Design review of the part built by this model. Coordinates are the model's own, in mm. A direction names the side the tool comes from. Round coordinates to 2 decimals unless told otherwise and drop trailing zeros. Loops run counter-clockwise (first coordinate to the right, second up) from the corner with the lowest first, then second, coordinate; pieces in that order, holes last. Notation, with made-up numbers: (-28, 9) - (16, 9) arc R25 ccw to (16, 34) - close; hole circle Ø11 at (68, 51). An arc over 180 degrees is marked (long way). Return JSON: item names as keys, results as strings. Group by question number.
(1) We need section A-A, the plane z = 0.75. Write out the cut boundary in (x, y).
(2) Wall thickness on L1, parallel to X at y = 0, z = 4.5; L2, parallel to X at y = 0.85, z = 5.75; L3, parallel to Z at x = 1.9, y = 1.45: over which ranges is each line inside the solid? List them lowest first. Write a range as [from, to].
(3) For faces 5 (the cylindrical face through (1.03, -0.23, 3.95)), 6 (the cylindrical face through (-0.17, -1.29, 8.46)), 7 (the flat face through (-0.04, -1.24, 0)), list the 3-axis set-ups (+Z, -Z, +X, -X, +Y, -Y) from which the entire face can be reached by the end or side of a thin tool; tool diameter is ignored.
(4) We need section C-C, the plane x = 1.65. Write out the cut boundary in (y, z), and give its area (3 significant figures).
(5) We need section B-B, the plane y = 2.3. Write out the cut boundary in (x, z), and give its area (3 significant figures).
(6) The part is to be moulded in two halves that separate along Y. For faces 1 (the flat face through (-1.233, -2.175, 2.958)), 2 (the flat face through (-1.267, 2.155, 2.958)), 3 (the conical face through (-0.112, -0.146, 8.325)), 4 (the flat face through (-2.5, 0, 3)), say which applies: pulls with the +Y half, pulls with the -Y half, needs draft (parallel to the pull), parting line crosses it, or undercut.
(7) Clearance check with flat-ended pins moving along their axes: pin 1 (1.5 mm diameter, centred on x = -1.5, z = 3, fed in from -Y); pin 2 (1.5 mm diameter, centred on x = 0, z = 10, fed in from -Y); pin 3 (1.7 mm diameter, centred on x = 0, y = 0, fed in from -Z). State where each tip first meets the part, or that it passes through.
Autodesk Inventor part; units mm, degrees
ref_plane "YZ Plane" through (0, 0, 0) normal (1, 0, 0) x (0, 1, 0)
ref_plane "XZ Plane" through (0, 0, 0) normal (0, 1, 0) x (-1, 0, 0)
ref_plane "XY Plane" through (0, 0, 0) normal (0, 0, 1) x (1, 0, 0)
sketch "スケッチ1" plane through (0, 0, 0) normal (0, 0, 1) x (1, 0, 0)
  line L0 (0, 2.8868) -> (2.5, 1.4434)
  line L1 (2.5, 1.4434) -> (2.5, -1.4434)
  line L2 (2.5, -1.4434) -> (0, -2.8868)
  line L3 (0, -2.8868) -> (-2.5, -1.4434)
  line L4 (-2.5, -1.4434) -> (-2.5, 1.4434)
  line L5 (-2.5, 1.4434) -> (0, 2.8868)
  point P0 (0, 0)
  point P1 (0, 0)
  dimension "d0" = 5
extrude "押し出し1" add sketch "スケッチ1" along normal blind 6
sketch "スケッチ2" plane through (0, 0, 6) normal (0, 0, 1) x (1, 0, 0)
  circle A0 centre (0, 0) radius 1.3
  dimension "d3" = 2.6
extrude "押し出し2" add sketch "スケッチ2" along normal blind 5
thread "ねじ1"
sketch "スケッチ3" plane through (0, 0, 0) normal (0, 0, -1) x (-1, 0, 0)
  point P0 (0, 0)
hole "穴1" at (0, 0, 0) direction (0, 0, 1) diameter 2.113 depth 7.8 tip angle 118
properties part number "ジュラコンスペーサー（六角）_BS-2606E" material "アセタール樹脂、白"
Solutions:
{
 "1": {"outline": "(-2.5, -1.44) - (0, -2.89) - (2.5, -1.44) - (2.5, 1.44) - (0, 2.89) - (-2.5, 1.44) - close; hole circle Ø2.11 at (0, 0)"},
 "2": {"L1": "[-2.5, -1.06], [1.06, 2.5]", "L2": "[-2.5, -0.63], [0.63, 2.5]", "L3": "[0, 6]"},
 "3": {"face 5": "-Z", "face 6": "+Z", "face 7": "-Z, +X, -X, +Y, -Y"},
 "4": {"outline": "(-1.93, 0) - (1.93, 0) - (1.93, 6) - (-1.93, 6) - close", "area": "23.2 mm^2"},
 "5": {"outline": "(-1.02, 0) - (1.02, 0) - (1.02, 6) - (-1.02, 6) - close", "area": "12.2 mm^2"},
 "6": {"face 1": "pulls with the -Y half", "face 2": "pulls with the +Y half", "face 3": "undercut", "face 4": "needs draft"},
 "7": {"pin 1": "y = -2.45", "pin 2": "y = -1.3", "pin 3": "z = 7.92"}
}
